For this review, take the finished solid that the model builds, in its own axes (mm). Give positions to 0.01 mm unless a question says otherwise; leave off trailing zeros. Answer as CSV lines item,"result".
```python
from build123d import *

# Parameters (mm, degrees)
SKETCH1_W                 = 60
SKETCH1_H                 = 45
BOSS_EXTRUDE1_DEPTH       = 2
F_3_0MM_DOWEL_HOLE1_D     = 3
F_3_0MM_DOWEL_HOLE1_DEPTH = 20
F_3_0MM_DOWEL_HOLE1_TIP   = 0.901290929
FILLET2_R                 = 1
FILLET1_R                 = 1


with BuildPart() as part:
    # Sketch1 → Boss-Extrude1 (new body)
    with BuildSketch(Plane(origin=(0, 0, 0), x_dir=(0, 0, -1), z_dir=(1, 0, 0))):
        Rectangle(SKETCH1_W, SKETCH1_H)
    extrude(amount=BOSS_EXTRUDE1_DEPTH)

    # Ø3.0mm Dowel Hole1
    with Locations(Plane(origin=(2, 0, 0), x_dir=(0, 0, -1), z_dir=(1, 0, 0))):
        with Locations((-27.5, 20), (27.5, 20), (27.5, -20), (-27.5, -20)):
            Hole(F_3_0MM_DOWEL_HOLE1_D / 2, depth=F_3_0MM_DOWEL_HOLE1_DEPTH)
            with Locations((0, 0, -(F_3_0MM_DOWEL_HOLE1_DEPTH + F_3_0MM_DOWEL_HOLE1_TIP / 2))):  # 118° drill point
                Cone(0, F_3_0MM_DOWEL_HOLE1_D / 2, F_3_0MM_DOWEL_HOLE1_TIP, mode=Mode.SUBTRACT)

    # Fillet2
    fillet2_edges = [part.edges().sort_by_distance(p)[0] for p in [
        (1, -22.5, -30),
        (1, -22.5, 30),
        (1, 22.5, 30),
        (1, 22.5, -30),
    ]]
    fillet(fillet2_edges, radius=FILLET2_R)

    # Fillet1
    fillet1_edges = [part.edges().sort_by_distance(p)[0] for p in [
        (2, 0, -30),
        (2, -22.5, 0),
        (2, 22.5, 0),
        (2, 0, 30),
        (2, 22.207106781, 29.707106781),
        (2, 22.207106781, -29.707106781),
        (2, -22.207106781, 29.707106781),
        (2, -22.207106781, -29.707106781),
    ]]
    fillet(fillet1_edges, radius=FILLET1_R - 0.0001)  # a hair under: the kernel refuses the full size


solid = part.part
```
Q1. Clearance check with flat-ended pins moving along their axes: pin 1 (6 mm diameter, centred on y = 16.5, z = -2.5, fed in from -X); pin 2 (1.8 mm diameter, centred on y = -20, z = -27.5, fed in from -X). State where each tip first meets the part, or that it passes through.
Answer block:
pin 1,"stops at x = 0"
pin 2,"passes through"
Q2. Draft analysis for pull direction Z (two halves, no side actions). For faces 1 (the flat face through (2, 0, 0)), 2 (the cylindrical face through (0.99, 21.01, -28.61)), state which applies: released by +Z, released by -Z, zero draft, split by the parting line, or undercut.
Answer block:
face 1,"zero draft"
face 2,"undercut"
Q3. Add section A-A (z = 27.5). State how many separate pieces and enclosed holes the cut face has, plus the area to 3 significant figures.
Answer block:
separate pieces,"3"
enclosed holes,"0"
area,"77.6 mm2"
Q4. To check wall thickness, follow probe 1 along Y at (x, z) = (0.8, 27.5); probe 2 along Y at (x, z) = (1.65, 27.5); probe 3 along Z at (x, y) = (1.7, 19). State the ranges of each line that lie inside material, in increasing order. Write a range as [from, to].
Answer block:
probe 1,"y = [-22.5, -21.5], [-18.5, 18.5], [21.5, 22.5]"
probe 2,"y = [-22.26, -21.5], [-18.5, 18.5], [21.5, 22.26]"
probe 3,"z = [-29.71, -28.62], [-26.38, 26.38], [28.62, 29.71]"
